from build123d import *

# Parameters (mm, degrees)
F0_W     = 76.2
F0_H     = 76.2
F1_DEPTH = 76.2
F3_R     = 6.35
F4_T     = 6.35


# Not quite as in the source:
# - a shell that OpenCascade refuses in one call is made with other operations: the cavity is built on its own and cut out


with BuildPart() as f1:
    # F0 (on Front) → F1 (new body)
    with BuildSketch(Plane.XZ):
        with Locations((-38.1, 38.1)):
            Rectangle(F0_W, F0_H)
    extrude(amount=F1_DEPTH)

    # F0 (on Front) → F2 (revolve)
    with BuildSketch(Plane.XZ):
        with Locations((-38.1, 38.1)):
            Rectangle(F0_W, F0_H)
    revolve(axis=Axis((0, 0, 38.1), (0, 0, 1)))

    # F3
    f3_edges = [f1.edges().sort_by_distance(p)[0] for p in [
        (-76.2, -38.1, 76.2),
        (-76.2, -76.2, 38.1),
    ]]
    fillet(f3_edges, radius=F3_R)

    # F4: shell of thickness 6.35, made by hand


with BuildPart() as f4_core1:
    # F4_t2: copy of F1
    add(f1.part)

    # the walls: a layer under each face that stays
    f4_faces = [f4_core1.faces().sort_by_distance(p)[0] for p in [
        (-34.925, -76.2, 34.925),
        (53.8815367264, 53.8815367264, 34.925),
        (-76.2, -34.925, 34.925),
        (0, 0, 76.2),
    ]]
    thicken(f4_faces, amount=-F4_T, mode=Mode.SUBTRACT)


with BuildPart() as f1_1:
    add(f1.part)

    # what is left inside the walls is the cavity
    f4_cavity = [f4_core1.part.solids().sort_by_distance(p)[0] for p in [
        (49.346507, 49.346507, 46.566667),
    ]]
    add(f4_cavity, mode=Mode.SUBTRACT)


solid = f1_1.part
The model under review builds one solid part; all positions refer to its coordinate system, in mm. A direction names the side the tool comes from. Give positions to 0.01 mm unless a question says otherwise; leave off trailing zeros. Order: outer loops, then holes, each group sorted by start corner. A loop starts at its lowest first (then second) coordinate and runs counter-clockwise, first axis right, second up. Notation, with made-up numbers: M 7.25,-28.75 L 22.25,-28.75 A17 cw 22.25,-14.75 Z; hole C -24,16.5 d3. An arc over 180 degrees is marked long. One line per question, with ' | ' between items. Start each with the question number.
1) Wall thickness on L1, parallel to Y at x = 0, z = 34; L2, parallel to Z at x = -49, y = 50; L3, parallel to Z at x = -18.5, y = -27: over which ranges is each line inside the solid? List them lowest first. Write a range as from..to.
2) Consider section A-A, the plane z = 45.5. Give the boundary of the cut face in (x, y).
3) Mouldability with a two-part tool opening along Y and no side actions: class faces 1 (the face through (1, -1, 69.85)), 2 (the face through (50.99, 47.74, 35.41)), 3 (the face through (-68, 17, 0)), 4 (the face through (55.629, 52.075, 35.414)) as pulls with the +Y half, pulls with the -Y half, needs draft (parallel to the pull), parting line crosses it, or undercut.
4) Clearance check with flat-ended pins moving along their axes: P1, Ø4, axis at x = 27.5, z = 66, coming from the -Y side; P2, Ø1, axis at y = 60.5, z = 49.5, coming from the -X side; P3, Ø21, axis at y = -44, z = 48.5, coming from the +X side. State where each tip first meets the part, or that it passes through.
5) For faces 5 (the face through (-35, -69.85, 35)), 6 (the face through (-74.39, -35.41, 74.29)), list the 3-axis set-ups (+Z, -Z, +X, -X, +Y, -Y) from which the entire face can be reached by the end or side of a thin tool; tool diameter is ignored.
Found:
1) L1: y = -76.2..-69.85, 69.85..76.2 | L2: z = 0..76.2 | L3: z = 69.85..76.2
2) outline: M -76.2,-69.85 A6.35 ccw -69.85,-76.2 L 0,-76.2 A76.2 ccw long -76.2,0 Z; hole M -69.85,-69.85 L 0,-69.85 A69.85 ccw long -69.85,0 Z
3) face 1: undercut | face 2: undercut | face 3: needs draft | face 4: parting line crosses it
4) P1: stops at y = -71.81 | P2: stops at x = -46.97 | P3: stops at x = 68.44
5) face 5: -Z | face 6: +Z, -X, +Y, -Y
